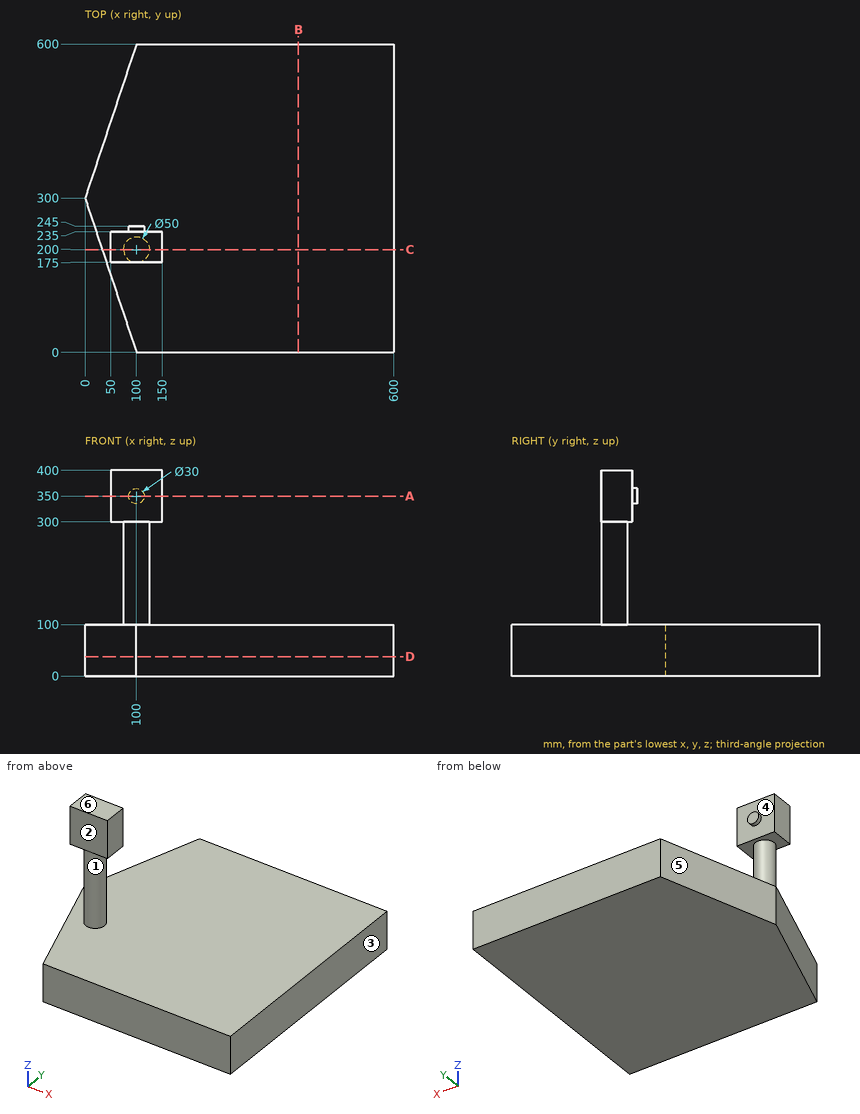
Here's the drawing with two shaded views (mm, measured from the low corner). I have some questions. A direction names the side the tool comes from. Round coordinates to 2 decimals unless told otherwise and drop trailing zeros. Order: outer loops, then holes, each group sorted by start corner. A loop starts at its lowest first (then second) coordinate and runs counter-clockwise, first axis right, second up. Notation, with made-up numbers: (49, 27) -> (83, 27) arc R18 cw to (83, 51) -> close; hole circle Ø3 at (45, 22). An arc over 180 degrees is marked (long way). Use a Markdown table: item, result. Add a question column.
(1) Suppose I cut it at B-B, the plane x = 415. Please give me the cut outline in (y, z), and give its area (3 significant figures).
(2) Suppose I cut it at C-C, the plane y = 200. Please give me the cut outline in (x, z).
(3) For pin 1 Ø12 at (x, y) = (409, 93.5) entering from +Z; pin 2 Ø24 at (x, z) = (98.5, 349.5) entering from +Y, each with a flat end and sliding along its axis, tell me the tip position at first contact or that it passes through.
(4) For the marked faces 1, 2 and 3, which set-ups out of +Z, -Z, +X, -X, +Y, -Y let a thin tool reach every point of the face, with its end or its side?
(5) Suppose I cut it at D-D, the plane z = 37.5. Please give me the cut outline in (x, y).
(6) Suppose I cut it at A-A, the plane z = 350. Please give me the cut outline in (x, y).
(7) I need wall thicknesses on line 1 along Z through (x, y) = (161, 154); line 2 along X through (y, z) = (156, 78.5); line 3 along X through (y, z) = (323.5, 70). Which ranges of each line are inside material? Lowest first, please.
(8) If we mould it in two halves opening along Z, with no side actions, what happens to the marked faces 4, 5 and 6? For each: released by +Z, released by -Z, zero draft, split by the parting line, or undercut.
Verdict:
| question | item | result |
|---|---|---|
| 1 | outline | (0, 0) -> (600, 0) -> (600, 100) -> (0, 100) -> close |
| 1 | area | 60,000 mm2 |
| 2 | outline | (33.33, 0) -> (600, 0) -> (600, 100) -> (125, 100) -> (125, 300) -> (150, 300) -> (150, 400) -> (50, 400) -> (50, 300) -> (75, 300) -> (75, 100) -> (33.33, 100) -> close |
| 3 | pin 1 | z = 100 |
| 3 | pin 2 | y = 245 |
| 4 | face 1 | none |
| 4 | face 2 | +Z, +X, -X, -Y |
| 4 | face 3 | +Z, -Z, +X, +Y, -Y |
| 5 | outline | (0, 300) -> (100, 0) -> (600, 0) -> (600, 600) -> (100, 600) -> close |
| 6 | outline | (50, 175) -> (150, 175) -> (150, 235) -> (115, 235) -> (115, 245) -> (85, 245) -> (85, 235) -> (50, 235) -> close |
| 7 | line 1 | 0 to 100 |
| 7 | line 2 | 48 to 600 |
| 7 | line 3 | 7.83 to 600 |
| 8 | face 4 | undercut |
| 8 | face 5 | zero draft |
| 8 | face 6 | released by +Z |
